from build123d import *

# Parameters (mm, degrees)
SKETCH1_W               = 60.96
SKETCH1_H               = 50.8
BOSS_EXTRUDE1_DEPTH     = 1.27
SKETCH2_W               = 11.43
SKETCH2_H               = 11.43
CUT_EXTRUDE1_DEPTH      = 2.27
FILLET2_R               = 1.27
SKETCH4_R               = 0.762
BOSS_EXTRUDE2_DEPTH     = 2.032
FILLET3_R               = 1.27
LPATTERN13_COUNT        = 4
LPATTERN13_PITCH        = 12.7
LPATTERN13_COUNT_DIR2   = 3
LPATTERN13_PITCH_DIR2   = 12.7
FILLET2_OF_LPATTERN13_R = 1.27
LPATTERN14_COUNT        = 3
LPATTERN14_PITCH        = 26.289
LPATTERN14_COUNT_DIR2   = 3
LPATTERN14_PITCH_DIR2   = 39.878


with BuildPart() as part:
    # Sketch1 → Boss-Extrude1 (new body)
    with BuildSketch(Plane(origin=(0, 0, 0), x_dir=(1, 0, 0), z_dir=(0, 1, 0))):
        Rectangle(SKETCH1_W, SKETCH1_H)
    extrude(amount=BOSS_EXTRUDE1_DEPTH)

    # Sketch2 → Cut-Extrude1 (cut, through all)
    with BuildSketch(Plane(origin=(0, 1.27, 0), x_dir=(1, 0, 0), z_dir=(0, 1, 0))):
        with Locations((-19.05, 12.7)):
            Rectangle(SKETCH2_W, SKETCH2_H)
    cut_extrude1 = extrude(amount=-CUT_EXTRUDE1_DEPTH, mode=Mode.SUBTRACT)

    # Fillet2
    fillet2_edges = [part.edges().sort_by_distance(p)[0] for p in [
        (-13.335, 0.635, -18.415),
        (-13.335, 0.635, -6.985),
        (-24.765, 0.635, -6.985),
        (-24.765, 0.635, -18.415),
    ]]
    fillet(fillet2_edges, radius=FILLET2_R)

    # Sketch4 → Boss-Extrude2 (add)
    with BuildSketch(Plane(origin=(0, 1.27, 0), x_dir=(1, 0, 0), z_dir=(0, 1, 0))):
        with Locations((-26.289, 19.939)):
            Circle(SKETCH4_R)
    boss_extrude2 = extrude(amount=BOSS_EXTRUDE2_DEPTH)

    # Fillet3
    fillet3_edges = [part.edges().sort_by_distance(p)[0] for p in [
        (-30.48, 0.635, -25.4),
        (30.48, 0.635, -25.4),
        (30.48, 0.635, 25.4),
        (-30.48, 0.635, 25.4),
    ]]
    fillet(fillet3_edges, radius=FILLET3_R)

    # LPattern13: Cut-Extrude1 4 × 3
    with Locations(*[(i * LPATTERN13_PITCH, 0, j * LPATTERN13_PITCH_DIR2) for i in range(LPATTERN13_COUNT) for j in range(LPATTERN13_COUNT_DIR2) if (i, j) != (0, 0)]):
        add(cut_extrude1, mode=Mode.SUBTRACT)

    # Fillet2 of LPattern13
    fillet2_of_lpattern13_edges = [part.edges().sort_by_distance(p)[0] for p in [
        (-13.335, 0.635, -5.715),
        (-13.335, 0.635, 5.715),
        (-24.765, 0.635, 5.715),
        (-24.765, 0.635, -5.715),
        (-13.335, 0.635, 6.985),
        (-13.335, 0.635, 18.415),
        (-24.765, 0.635, 18.415),
        (-24.765, 0.635, 6.985),
        (-0.635, 0.635, -18.415),
        (-0.635, 0.635, -6.985),
        (-12.065, 0.635, -6.985),
        (-12.065, 0.635, -18.415),
        (-0.635, 0.635, -5.715),
        (-0.635, 0.635, 5.715),
        (-12.065, 0.635, 5.715),
        (-12.065, 0.635, -5.715),
        (-0.635, 0.635, 6.985),
        (-0.635, 0.635, 18.415),
        (-12.065, 0.635, 18.415),
        (-12.065, 0.635, 6.985),
        (12.065, 0.635, -18.415),
        (12.065, 0.635, -6.985),
        (0.635, 0.635, -6.985),
        (0.635, 0.635, -18.415),
        (12.065, 0.635, -5.715),
        (12.065, 0.635, 5.715),
        (0.635, 0.635, 5.715),
        (0.635, 0.635, -5.715),
        (12.065, 0.635, 6.985),
        (12.065, 0.635, 18.415),
        (0.635, 0.635, 18.415),
        (0.635, 0.635, 6.985),
        (24.765, 0.635, -18.415),
        (24.765, 0.635, -6.985),
        (13.335, 0.635, -6.985),
        (13.335, 0.635, -18.415),
        (24.765, 0.635, -5.715),
        (24.765, 0.635, 5.715),
        (13.335, 0.635, 5.715),
        (13.335, 0.635, -5.715),
        (24.765, 0.635, 6.985),
        (24.765, 0.635, 18.415),
        (13.335, 0.635, 18.415),
        (13.335, 0.635, 6.985),
    ]]
    fillet(fillet2_of_lpattern13_edges, radius=FILLET2_OF_LPATTERN13_R)

    # LPattern14: Boss-Extrude2 3 × 3, 3 skipped
    with Locations(*[(i * LPATTERN14_PITCH, 0, j * LPATTERN14_PITCH_DIR2) for i in range(LPATTERN14_COUNT) for j in range(LPATTERN14_COUNT_DIR2) if (i, j) not in ((0, 0), (0, 2), (1, 2), (2, 2))]):
        add(boss_extrude2)


solid = part.part
Work out the finished part from the listing and answer in its coordinate system (mm). A direction names the side the tool comes from. Round coordinates to 2 decimals unless told otherwise and drop trailing zeros. Loops run counter-clockwise (first coordinate to the right, second up) from the corner with the lowest first, then second, coordinate; pieces in that order, holes last. Notation, with made-up numbers: (-24, 16.25) - (18, 16.25) arc R22 ccw to (18, 23.25) - close; hole circle Ø6 at (15.25, 51.25). An arc over 180 degrees is marked (long way). One line per item, written item: value.
Q1. Find section B-B on x = 16. Give the vertices of the cut face in (y, z) (3 decimals).
Check values:
outline: (0, -25.4) - (1.27, -25.4) - (1.27, -18.415) - (0, -18.415) - close; (0, -6.985) - (1.27, -6.985) - (1.27, -5.715) - (0, -5.715) - close; (0, 5.715) - (1.27, 5.715) - (1.27, 6.985) - (0, 6.985) - close; (0, 18.415) - (1.27, 18.415) - (1.27, 25.4) - (0, 25.4) - close
Q2. Straight lines are drawn through the part: probe 1 along X at (y, z) = (1, 16.5) (3 decimals); probe 2 along Z at (x, y) = (-5.5, 0.6) (3 decimals); probe 3 along X at (y, z) = (0.4, 18). For each, find the intervals that lie inside material, in ascending order.
Check values:
probe 1: -30.48 to -24.765, -13.335 to -12.065, -0.635 to 0.635, 12.065 to 13.335, 24.765 to 30.48
probe 2: -25.4 to -18.415, -6.985 to -5.715, 5.715 to 6.985, 18.415 to 25.4
probe 3: -30.48 to -24.43, -13.67 to -11.73, -0.97 to 0.97, 11.73 to 13.67, 24.43 to 30.48
Q3. The mould has two halves that part along X. Classify faces 1 (the flat face through (0, 3.302, -20)), 2 (the cylindrical face through (-24.383, 0.626, 5.353)): +X half, -X half, draft (parallel to the pull), parting line (faces both ways), or undercut.
Check values:
face 1: draft
face 2: undercut
Q4. For faces 3 (the cylindrical face through (-0.099, 2.272, 19.183)), 4 (the flat face through (-24.765, 1, 0)), determine the directions among +Z, -Z, +X, -X, +Y, -Y from which every point of the face is accessible in a straight line to the end or side of a thin tool.
Check values:
face 3: +Y
face 4: +Y, -Y
Q5. Find section C-C on y = 2.15. Give the vertices of the cut face in (x, z).
Check values:
outline: circle Ø1.52 at (-26.29, -19.94); circle Ø1.52 at (-26.29, 19.94); circle Ø1.52 at (0, -19.94); circle Ø1.52 at (0, 19.94); circle Ø1.52 at (26.29, -19.94); circle Ø1.52 at (26.29, 19.94)
Q6. Find section A-A on z = 3. Give the vertices of the cut face in (x, y) (3 decimals), and give its area (3 significant figures).
Check values:
outline: (-30.48, 0) - (-24.765, 0) - (-24.765, 1.27) - (-30.48, 1.27) - close; (-13.335, 0) - (-12.065, 0) - (-12.065, 1.27) - (-13.335, 1.27) - close; (-0.635, 0) - (0.635, 0) - (0.635, 1.27) - (-0.635, 1.27) - close; (12.065, 0) - (13.335, 0) - (13.335, 1.27) - (12.065, 1.27) - close; (24.765, 0) - (30.48, 0) - (30.48, 1.27) - (24.765, 1.27) - close
area: 19.4 mm2
